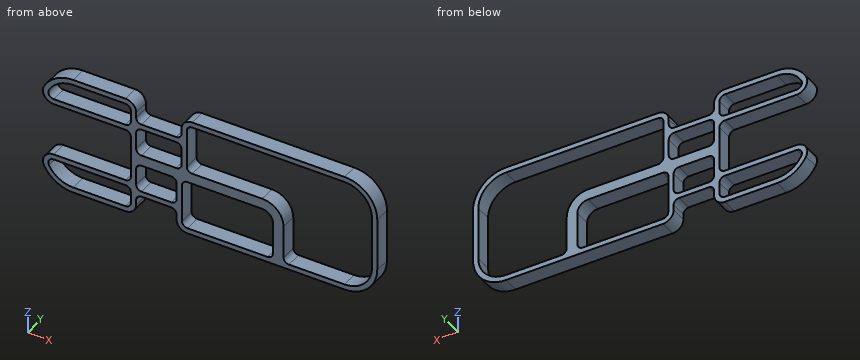
```python
from build123d import *

# Parameters (mm, degrees)
BOSS_EXTRUDE1_DEPTH   = 19.05
BOSS_EXTRUDE1_2_DEPTH = 19.05
SKETCH4_W             = 6.35
SKETCH4_H             = 63.131908364
CUT_EXTRUDE4_DEPTH    = 19.05
BOSS_EXTRUDE2_DEPTH   = 19.05
BOSS_EXTRUDE3_DEPTH   = 19.05
FILLET2_R             = 6.35
FILLET3_R             = 12.7
FILLET4_R             = 12.7
FILLET5_R             = 25.4


with BuildPart() as part:
    # Sketch1 → Boss-Extrude1 (new body)
    with BuildSketch(Plane(origin=(0, 0, 0), x_dir=(1, 0, 0), z_dir=(0, 1, 0))):
        with BuildLine():
            Line((-200.920268311, 32.916976578), (-200.920268311, -30.214931786))
            ThreePointArc((-200.920268311, -30.214931786), (-189.456017676, -57.892081151), (-161.778868311, -69.356331786))
            Line((-161.778868311, -69.356331786), (-86.620268311, -69.356331786))
            Line((-86.620268311, -69.356331786), (-86.620268311, -63.006331786))
            Line((-86.620268311, -63.006331786), (-161.778868311, -63.006331786))
            ThreePointArc((-161.778868311, -63.006331786), (-184.965889616, -53.401953091), (-194.570268311, -30.214931786))
            Line((-194.570268311, -30.214931786), (-194.570268311, 32.916976578))
            ThreePointArc((-194.570268311, 32.916976578), (-184.965889616, 56.103997883), (-161.778868311, 65.708376578))
            Line((-161.778868311, 65.708376578), (-86.620268311, 65.708376578))
            Line((-86.620268311, 65.708376578), (-86.620268311, 72.058376578))
            Line((-86.620268311, 72.058376578), (-161.778868311, 72.058376578))
            ThreePointArc((-161.778868311, 72.058376578), (-189.456017676, 60.594125943), (-200.920268311, 32.916976578))
        make_face()
    extrude(amount=BOSS_EXTRUDE1_DEPTH)

    # Sketch4 → Cut-Extrude4 (cut)
    with BuildSketch(Plane(origin=(0, 19.05, 0), x_dir=(1, 0, 0), z_dir=(0, 1, 0))):
        with Locations((-197.745268311, 1.351022396)):
            Rectangle(SKETCH4_W, SKETCH4_H)
    extrude(amount=-CUT_EXTRUDE4_DEPTH, mode=Mode.SUBTRACT)

    # Sketch5 → Boss-Extrude2 (add)
    with BuildSketch(Plane(origin=(0, 0, 0), x_dir=(1, 0, 0), z_dir=(0, 1, 0))):
        with BuildLine():
            Line((-194.570268311, -30.214931786), (-86.620268311, -30.214931786))
            Line((-86.620268311, -30.214931786), (-86.620268311, -63.006331786))
            Line((-86.620268311, -63.006331786), (-92.970268311, -63.006331786))
            Line((-92.970268311, -63.006331786), (-92.970268311, -36.564931786))
            Line((-92.970268311, -36.564931786), (-193.949560159, -36.564931786))
            ThreePointArc((-193.949560159, -36.564931786), (-194.414722357, -33.405064174), (-194.570268311, -30.214931786))
        make_face()
        with BuildLine():
            Line((-92.970268311, 65.708376578), (-86.620268311, 65.708376578))
            Line((-86.620268311, 65.708376578), (-86.620268311, 32.916976578))
            Line((-86.620268311, 32.916976578), (-194.570268311, 32.916976578))
            ThreePointArc((-194.570268311, 32.916976578), (-194.414722357, 36.107108966), (-193.949560159, 39.266976578))
            Line((-193.949560159, 39.266976578), (-92.970268311, 39.266976578))
            Line((-92.970268311, 39.266976578), (-92.970268311, 65.708376578))
        make_face()
    extrude(amount=BOSS_EXTRUDE2_DEPTH)



with BuildPart() as body_2:
    # Sketch1 → Boss-Extrude1 2 (new body)
    with BuildSketch(Plane(origin=(0, 0, 0), x_dir=(1, 0, 0), z_dir=(0, 1, 0))):
        with BuildLine():
            Line((200.844440053, -30.214931786), (200.844440053, 32.916976578))
            ThreePointArc((200.844440053, 32.916976578), (189.380189418, 60.594125943), (161.703040053, 72.058376578))
            Line((161.703040053, 72.058376578), (-38.360268311, 72.058376578))
            Line((-38.360268311, 72.058376578), (-38.360268311, 65.708376578))
            Line((-38.360268311, 65.708376578), (161.703040053, 65.708376578))
            ThreePointArc((161.703040053, 65.708376578), (184.890061358, 56.103997883), (194.494440053, 32.916976578))
            Line((194.494440053, 32.916976578), (194.494440053, -30.214931786))
            ThreePointArc((194.494440053, -30.214931786), (184.890061358, -53.401953091), (161.703040053, -63.006331786))
            Line((161.703040053, -63.006331786), (-32.518268311, -63.006331786))
            Line((-32.518268311, -63.006331786), (-32.518268311, -69.356331786))
            Line((-32.518268311, -69.356331786), (161.703040053, -69.356331786))
            ThreePointArc((161.703040053, -69.356331786), (189.380189418, -57.892081151), (200.844440053, -30.214931786))
        make_face()
    extrude(amount=BOSS_EXTRUDE1_2_DEPTH)


with BuildPart() as part_1:
    add(part.part)

    add(body_2.part)  # Boss-Extrude3 merges body 2
    # Sketch6 → Boss-Extrude3 (add)
    with BuildSketch(Plane(origin=(0, 0, 0), x_dir=(1, 0, 0), z_dir=(0, 1, 0))):
        Polygon((-86.620268311, -43.956331786), (-32.518268311, -43.956331786), (-32.518268311, -63.006331786), (-26.168268311, -63.006331786), (-26.168268311, -37.606331786), (-26.168268311, -4.998977604), (89.084440053, -4.998977604), (89.084440053, 65.708376578), (76.384440053, 65.708376578), (76.384440053, 7.701022396), (-32.010268311, 7.701022396), (-32.010268311, 40.308376578), (-32.010268311, 65.708376578), (-38.360268311, 65.708376578), (-38.360268311, 46.658376578), (-86.620268311, 46.658376578), (-86.620268311, 40.308376578), (-38.360268311, 40.308376578), (-38.360268311, 7.701022396), (-86.620268311, 7.701022396), (-86.620268311, 32.916976578), (-92.970268311, 32.916976578), (-92.970268311, 7.701022396), (-92.970268311, -4.998977604), (-92.970268311, -30.214931786), (-86.620268311, -30.214931786), (-86.620268311, -4.998977604), (-32.518268311, -4.998977604), (-32.518268311, -37.606331786), (-86.620268311, -37.606331786), align=None)
    extrude(amount=BOSS_EXTRUDE3_DEPTH)

    # Fillet2
    fillet2_edges = [part_1.edges().sort_by_distance(p)[0] for p in [
        (-193.949560159, 9.525, 36.564931786),
        (-92.970268311, 9.525, 36.564931786),
        (-193.949560159, 9.525, -39.266976578),
        (-92.970268311, 9.525, -65.708376578),
        (-92.970268311, 9.525, -39.266976578),
        (-86.620268311, 9.525, 37.606331786),
        (-86.620268311, 9.525, 43.956331786),
        (-32.518268311, 9.525, 43.956331786),
        (-26.168268311, 9.525, 63.006331786),
        (-26.168268311, 9.525, 4.998977604),
        (89.084440053, 9.525, -65.708376578),
        (76.384440053, 9.525, -65.708376578),
        (-32.010268311, 9.525, -7.701022396),
        (-32.010268311, 9.525, -65.708376578),
        (-38.360268311, 9.525, -46.658376578),
        (-86.620268311, 9.525, -46.658376578),
        (-86.620268311, 9.525, -40.308376578),
        (-38.360268311, 9.525, -40.308376578),
        (-38.360268311, 9.525, -7.701022396),
        (-86.620268311, 9.525, -7.701022396),
        (-92.970268311, 9.525, -32.916976578),
        (-92.970268311, 9.525, 30.214931786),
        (-86.620268311, 9.525, 4.998977604),
        (-32.518268311, 9.525, 4.998977604),
        (-32.518268311, 9.525, 37.606331786),
        (-92.970268311, 9.525, 63.006331786),
    ]]
    fillet(fillet2_edges, radius=FILLET2_R)

    # Fillet3
    fillet3_edges = [part_1.edges().sort_by_distance(p)[0] for p in [
        (-200.920268311, 9.525, 30.214931786),
        (-200.920268311, 9.525, -32.916976578),
        (-86.620268311, 9.525, -72.058376578),
        (-32.518268311, 9.525, 69.356331786),
        (-38.360268311, 9.525, -72.058376578),
        (-86.620268311, 9.525, 69.356331786),
    ]]
    fillet(fillet3_edges, radius=FILLET3_R)

    # Fillet4
    fillet4_edges = [part_1.edges().sort_by_distance(p)[0] for p in [
        (76.384440053, 9.525, -7.701022396),
    ]]
    fillet(fillet4_edges, radius=FILLET4_R)

    # Fillet5
    fillet5_edges = [part_1.edges().sort_by_distance(p)[0] for p in [
        (89.084440053, 9.525, 4.998977604),
    ]]
    fillet(fillet5_edges, radius=FILLET5_R)


solid = part_1.part
```
Here's how the part is built. I have some questions about the finished solid (model axes, mm). Coordinates: 2 decimals unless noted, no trailing zeros. Write each loop counter-clockwise with the first axis right and the second up, starting at its lowest first coordinate (ties: lowest second). Pieces come first, ordered by that corner, then holes. Notation, with made-up numbers: M 81.5,56.5 L 140.5,56.5 A6 cw 140.5,65.5 Z; hole C 44.5,26 d11. An arc over 180 degrees is marked long. Answer as CSV lines item,"result". Start each with the question number.
Q1. Suppose I cut it at D-D, the plane y = 3.75. State how many separate pieces and enclosed holes the cut face has, then the cut area to 3 significant figures.
Q2. Suppose I cut it at B-B, the plane x = -116. List the corners of the cut face in (y, z) for me, then the cut area to 3 significant figures.
Q3. I need wall thicknesses on probe 1 along Z at (x, y) = (-146, 3.25); probe 2 along Z at (x, y) = (15, 10.5); probe 3 along Z at (x, y) = (-59, 14.5). Which ranges of each line are inside material? Lowest first, please. Write a range as [from, to].
Q4. Will these pins go through, and if not, where does the flat tip stop? pin 1 Ø3 at (y, z) = (10, 53.5) entering from -X; pin 2 Ø4 at (y, z) = (14, -40.5) entering from -X; pin 3 Ø4 at (y, z) = (8, 50) entering from -X; pin 4 Ø12 at (x, z) = (-100.5, -23.5) entering from +Y.
Q5. Suppose I cut it at C-C, the plane x = 150.5. List the corners of the cut face in (y, z) for me.
Q6. Suppose I cut it at A-A, the plane x = 21. List the corners of the cut face in (y, z) for me, then the cut area to 3 significant figures.
Entries:
1,separate pieces,"1"
1,enclosed holes,"6"
1,area,"11,600 mm²"
2,outline,"M 0,-72.06 L 19.05,-72.06 L 19.05,-65.71 L 0,-65.71 Z; M 0,-39.27 L 19.05,-39.27 L 19.05,-32.92 L 0,-32.92 Z; M 0,30.21 L 19.05,30.21 L 19.05,36.56 L 0,36.56 Z; M 0,63.01 L 19.05,63.01 L 19.05,69.36 L 0,69.36 Z"
2,area,"484 mm²"
3,probe 1,"z = [-72.06, -65.71], [-39.27, -32.92], [30.21, 36.56], [63.01, 69.36]"
3,probe 2,"z = [-72.06, -65.71], [-7.7, 5], [63.01, 69.36]"
3,probe 3,"z = [-46.66, -40.31], [-7.7, 5], [37.61, 43.96]"
4,pin 1,"stops at x = -194.3"
4,pin 2,"stops at x = -197.28"
4,pin 3,"stops at x = -196.61"
4,pin 4,"passes through"
5,outline,"M 0,-72.06 L 19.05,-72.06 L 19.05,-65.71 L 0,-65.71 Z; M 0,63.01 L 19.05,63.01 L 19.05,69.36 L 0,69.36 Z"
6,outline,"M 0,-72.06 L 19.05,-72.06 L 19.05,-65.71 L 0,-65.71 Z; M 0,-7.7 L 19.05,-7.7 L 19.05,5 L 0,5 Z; M 0,63.01 L 19.05,63.01 L 19.05,69.36 L 0,69.36 Z"
6,area,"484 mm²"
